The listing builds one solid part. Answer for the finished solid, in the listing's coordinates (mm). A direction names the side the tool comes from. Round coordinates to 2 decimals unless told otherwise and drop trailing zeros. Write each loop counter-clockwise with the first axis right and the second up, starting at its lowest first coordinate (ties: lowest second). Pieces come first, ordered by that corner, then holes. Notation, with made-up numbers: (-37.5, -19.75) - (-27.5, -19.75) arc R21 cw to (-27.5, 5.25) - close; hole circle Ø8 at (72.25, 36). An arc over 180 degrees is marked (long way). Return JSON: item names as keys, results as strings. Group by question number.
(1) Section C-C, the plane x = -1.7 is taken. Write down the section's boundary in (y, z), then the cut area to 3 significant figures.
(2) Each of these flat-tipped pins is pushed along its axis until it touches: pin 1 (1 mm diameter, centred on y = -1.5, z = -2, fed in from +X); pin 2 (1 mm diameter, centred on x = 0, z = -5, fed in from -Y); pin 3 (3 mm diameter, centred on x = -1, y = 0.5, fed in from -Z). Where does it stop, or does it pass through?
(3) Determine the mould class of faces 3 (the flat face through (0.76, 1.293, 1.961)), 4 (the flat face through (1.2, -1.2, 0)), 5 (the flat face through (0, 0, 1.2)), 6 (the cylindrical face through (-1.5, 0.07, -3.2)) for opening direction X: +X half, -X half, draft (parallel to the pull), parting line (faces both ways), or undercut.
(4) Section A-A, the plane z = 1.5 is taken. Write down the section's boundary in (x, y), then the cut area to 3 significant figures.
(5) Find the intervals of material crossed by line 1 along Z through (x, y) = (2.45, -0.4); line 2 along Y through (x, z) = (-0.8, 1.5); line 3 along X through (y, z) = (0.7, -3.75), in increasing order. Write a range as [from, to].
(6) Which of the six approach directions +Z, -Z, +X, -X, +Y, -Y give full straight-line access (tool end or side, diameter ignored) to faces 1 (the cylindrical face through (-0.596, -2.685, 1.331)), 2 (the flat face through (-0.74, 1.305, 1.961))?
(7) Section B-B, the plane z = -6.75 is taken. Write down the section's boundary in (x, y), then the cut area to 3 significant figures.
(8) Section D-D, the plane y = 2.15 is taken. Write down the section's boundary in (x, z).
```python
from build123d import *

# Parameters (mm, degrees)
F0_R     = 2.75
F0_R_2   = 1.5
F1_DEPTH = 2.7
F2_DEPTH = 8
F3_SIZE  = 1.5
F5_DEPTH = 1.5


with BuildPart() as f1:
    # F0 (on Top) → F1 (new body)
    with BuildSketch(Plane.XY):
        Circle(F0_R)
        Circle(F0_R_2, mode=Mode.SUBTRACT)
        Circle(F0_R_2)
    extrude(amount=F1_DEPTH)

    # F0 (on Top) → F2 (join)
    with BuildSketch(Plane.XY):
        Circle(F0_R_2)
    extrude(amount=-F2_DEPTH)

    # F3
    f3_edges = [f1.edges().sort_by_distance(p)[0] for p in [
        (-1.5, 0, -8),
    ]]
    chamfer(f3_edges, length=F3_SIZE)

    # F4 (on face) → F5 (cut)
    with BuildSketch(Plane.XY.offset(2.7)):
        Polygon((1.5, -0.866025), (1.5, 0.866025), (0, 1.732051), (-1.5, 0.866025), (-1.5, -0.866025), (0, -1.732051), align=None)
    extrude(amount=-F5_DEPTH, mode=Mode.SUBTRACT)


solid = f1.part
```
Working result:
{
 "1": {"outline": "(-2.16, 0) - (2.16, 0) - (2.16, 2.7) - (-2.16, 2.7) - close", "area": "11.7 mm^2"},
 "2": {"pin 1": "stops at x = 1.12", "pin 2": "stops at y = -1.5", "pin 3": "stops at z = -8"},
 "3": {"face 3": "undercut", "face 4": "draft", "face 5": "undercut", "face 6": "parting line"},
 "4": {"outline": "circle Ø5.5 at (0, 0); hole (-1.5, -0.87) - (0, -1.73) - (1.5, -0.87) - (1.5, 0.87) - (0, 1.73) - (-1.5, 0.87) - close", "area": "16.0 mm^2"},
 "5": {"line 1": "z = [0, 2.7]", "line 2": "y = [-2.63, -1.27], [1.27, 2.63]", "line 3": "x = [-1.33, 1.33]"},
 "6": {"face 1": "+Z, -Z", "face 2": "+Z"},
 "7": {"outline": "circle Ø2.5 at (0, 0)", "area": "4.91 mm^2"},
 "8": {"outline": "(-1.71, 0) - (1.71, 0) - (1.71, 2.7) - (-1.71, 2.7) - close"}
}
